Geometry check sheet. Reference: the model listing, model coordinates, mm. A direction names the side the tool comes from. Coordinates: 2 decimals unless noted, no trailing zeros. Order: outer loops, then holes, each group sorted by start corner. A loop starts at its lowest first (then second) coordinate and runs counter-clockwise, first axis right, second up. Notation, with made-up numbers: M 1,35 L 56,35 A19 ccw 56,54 Z; hole C 3,21.25 d9. An arc over 180 degrees is marked long. One line per item, written item: value. Start each with the question number.
1) Draft check along Z on faces 3 (the cylindrical face through (-2.522, 2.423, -48.156)), 4 (the flat face through (0, 2, 70.25)), 5 (the flat face through (-1, 2, -95.25)). Enter one of: pulls with the +Z half, pulls with the -Z half, needs draft (parallel to the pull), parting line crosses it, or undercut.
2) Sectioned sample at B-B, the plane x = -17. Enter the section's corners in (y, z).
3) Thickness scan on L1, parallel to X at y = 4.6, z = 73.5; L2, parallel to X at y = 0.4, z = -82.5; L3, parallel to Z at x = -28.5, y = 4.55. Record the ranges inside material, lowest first. Write a range as from..to.
4) Sectioned sample at A-A, the plane y = 2.7. State how many separate pieces and enclosed holes the cut face has, then the cut area to 3 significant figures.
5) Access from +Z, -Z, +X, -X, +Y, -Y to the whole of each face (thin tool, end or side, straight path). Record for faces 1 (the flat face through (-1, 0, -1)), 2 (the flat face through (32.28, 2, 83)).
```python
from build123d import *

# Parameters (mm, degrees)
SKETCH1_W           = 193.68
SKETCH1_H           = 190.5
BOSS_EXTRUDE1_DEPTH = 4.78
SKETCH2_R           = 2.6797
CUT_EXTRUDE1_DEPTH  = 5.78
CUT_EXTRUDE2_DEPTH  = 5.78
SKETCH4_R           = 1.936199963
SKETCH4_R_2         = 2.048699992
SKETCH4_R_3         = 1.9812
SKETCH4_R_4         = 2.038700012
CUT_EXTRUDE3_DEPTH  = 5.78


with BuildPart() as part:
    # Sketch1 → Boss-Extrude1 (new body)
    with BuildSketch(Plane(origin=(0, 0, 0), x_dir=(1, 0, 0), z_dir=(0, 1, 0))):
        Rectangle(SKETCH1_W, SKETCH1_H)
    extrude(amount=BOSS_EXTRUDE1_DEPTH)

    # Sketch2 → Cut-Extrude1 (cut, through all)
    with BuildSketch(Plane(origin=(0, 4.78, 0), x_dir=(1, 0, 0), z_dir=(0, 1, 0))):
        with Locations((0, 82.55)):
            Circle(SKETCH2_R)
    extrude(amount=-CUT_EXTRUDE1_DEPTH, mode=Mode.SUBTRACT)

    # Sketch3 → Cut-Extrude2 (cut, through all)
    with BuildSketch(Plane(origin=(0, 4.78, 0), x_dir=(1, 0, 0), z_dir=(0, 1, 0))):
        Polygon((0, -95.25), (-32.28, -95.25), (-32.28, -70.249999962), (32.28, -70.249999962), (32.28, -95.25), align=None)
    extrude(amount=-CUT_EXTRUDE2_DEPTH, mode=Mode.SUBTRACT)

    # Sketch4 → Cut-Extrude3 (cut, through all)
    with BuildSketch(Plane(origin=(0, 4.78, 0), x_dir=(1, 0, 0), z_dir=(0, 1, 0))):
        with Locations((10.5225, 56.962500062)):
            Circle(SKETCH4_R)
        with Locations((84.0775, 56.9625)):
            Circle(SKETCH4_R)
        with Locations((-38.005, 73.274999999)):
            Circle(SKETCH4_R_2)
        with Locations((-2.255, 73.275)):
            Circle(SKETCH4_R_2)
        with Locations((-2.255, 46.125)):
            Circle(SKETCH4_R_2)
        with Locations((-38.005, 46.125000001)):
            Circle(SKETCH4_R_2)
        with Locations((-83.8225, -41.381999999)):
            Circle(SKETCH4_R_3)
        with Locations((-83.822499999, 20.340000001)):
            Circle(SKETCH4_R_3)
        with Locations((-29.212499999, 20.34)):
            Circle(SKETCH4_R_3)
        with Locations((-29.2125, -41.382)):
            Circle(SKETCH4_R_3)
        with Locations((64.27, -20.864999962)):
            Circle(SKETCH4_R_4)
        with Locations((-9.61, -20.864999962)):
            Circle(SKETCH4_R_4)
    extrude(amount=-CUT_EXTRUDE3_DEPTH, mode=Mode.SUBTRACT)


solid = part.part
```
Final values:
1. face 3: undercut
1. face 4: pulls with the +Z half
1. face 5: pulls with the -Z half
2. outline: M 0,-95.25 L 4.78,-95.25 L 4.78,70.25 L 0,70.25 Z
3. L1: x = -96.84..-32.28, 32.28..96.84
3. L2: x = -96.84..-2.68, 2.68..96.84
3. L3: z = -95.25..-22.19, -18.49..39.53, 43.23..70.25
4. separate pieces: 1
4. enclosed holes: 13
4. area: 35,100 mm^2
5. face 1: +Z, -Z, +X, -X, -Y
5. face 2: +Z, +Y, -Y
